```python
from build123d import *

# Parameters (mm, degrees)
SKETCH1_W           = 25
SKETCH1_H           = 25
SKETCH1_W_2         = 23
SKETCH1_H_2         = 23
BOSS_EXTRUDE1_DEPTH = 450
SKETCH2_W           = 25
SKETCH2_H           = 25
SKETCH2_W_2         = 23
SKETCH2_H_2         = 23
BOSS_EXTRUDE2_DEPTH = 200
SKETCH3_W           = 25
SKETCH3_H           = 25
SKETCH3_W_2         = 23
SKETCH3_H_2         = 23
BOSS_EXTRUDE3_DEPTH = 200
SKETCH4_W           = 25
SKETCH4_H           = 25
SKETCH4_W_2         = 23
SKETCH4_H_2         = 23
BOSS_EXTRUDE4_DEPTH = 125
SKETCH5_W           = 25
SKETCH5_H           = 25
SKETCH5_W_2         = 23
SKETCH5_H_2         = 23
BOSS_EXTRUDE5_DEPTH = 50
SKETCH6_R           = 2
CUT_EXTRUDE1_DEPTH  = 25
SKETCH7_W           = 25
SKETCH7_H           = 25
SKETCH7_W_2         = 23
SKETCH7_H_2         = 23
BOSS_EXTRUDE6_DEPTH = 125
SKETCH8_W           = 25
SKETCH8_H           = 25
SKETCH8_W_2         = 23
SKETCH8_H_2         = 23
BOSS_EXTRUDE7_DEPTH = 400


with BuildPart() as part:
    # Sketch1 → Boss-Extrude1 (new body)
    with BuildSketch(Plane.XY):
        Rectangle(SKETCH1_W, SKETCH1_H)
        Rectangle(SKETCH1_W_2, SKETCH1_H_2, mode=Mode.SUBTRACT)
    boss_extrude1 = extrude(amount=BOSS_EXTRUDE1_DEPTH)

    # Sketch2 → Boss-Extrude2 (add)
    with BuildSketch(Plane(origin=(12.5, 0, 0), x_dir=(0, 0, -1), z_dir=(1, 0, 0))):
        with Locations((-437.5, 0)):
            Rectangle(SKETCH2_W, SKETCH2_H)
        with Locations((-437.5, 0)):
            Rectangle(SKETCH2_W_2, SKETCH2_H_2, mode=Mode.SUBTRACT)
    boss_extrude2 = extrude(amount=BOSS_EXTRUDE2_DEPTH)

    # Sketch3 → Boss-Extrude3 (add)
    with BuildSketch(Plane(origin=(12.5, 0, 0), x_dir=(0, 0, -1), z_dir=(1, 0, 0))):
        with Locations((-12.5, 0)):
            Rectangle(SKETCH3_W, SKETCH3_H)
        with Locations((-12.5, 0)):
            Rectangle(SKETCH3_W_2, SKETCH3_H_2, mode=Mode.SUBTRACT)
    boss_extrude3 = extrude(amount=BOSS_EXTRUDE3_DEPTH)

    # Mirror1: Boss-Extrude1, Boss-Extrude2, Boss-Extrude3 across plane
    add(boss_extrude1.mirror(Plane(origin=(212.5, 0, 0), x_dir=(0, 0, 1), z_dir=(1, 0, 0))))
    add(boss_extrude2.mirror(Plane(origin=(212.5, 0, 0), x_dir=(0, 0, 1), z_dir=(1, 0, 0))))
    add(boss_extrude3.mirror(Plane(origin=(212.5, 0, 0), x_dir=(0, 0, 1), z_dir=(1, 0, 0))))

    # Sketch4 → Boss-Extrude4 (add)
    with BuildSketch(Plane(origin=(0, 12.5, 0), x_dir=(1, 0, 0), z_dir=(0, 1, 0))):
        with Locations((425, -187.5)):
            Rectangle(SKETCH4_W, SKETCH4_H)
        with Locations((425, -187.5)):
            Rectangle(SKETCH4_W_2, SKETCH4_H_2, mode=Mode.SUBTRACT)
    extrude(amount=BOSS_EXTRUDE4_DEPTH)

    # Sketch5 → Boss-Extrude5 (add)
    with BuildSketch(Plane.ZY.offset(-412.5)):
        with Locations((187.5, 125)):
            Rectangle(SKETCH5_W, SKETCH5_H)
        with Locations((187.5, 125)):
            Rectangle(SKETCH5_W_2, SKETCH5_H_2, mode=Mode.SUBTRACT)
    extrude(amount=BOSS_EXTRUDE5_DEPTH)

    # Sketch6 → Cut-Extrude1 (cut)
    with BuildSketch(Plane(origin=(0, 137.5, 0), x_dir=(1, 0, 0), z_dir=(0, 1, 0))):
        with Locations(Location((367.5, -180, 0), (0, 0, 270))):
            Circle(SKETCH6_R)
        with Locations(Location((367.5, -195, 0), (0, 0, 270))):
            Circle(SKETCH6_R)
        with Locations(Location((377.5, -180, 0), (0, 0, 270))):
            Circle(SKETCH6_R)
        with Locations(Location((377.5, -195, 0), (0, 0, 270))):
            Circle(SKETCH6_R)
        with Locations(Location((387.5, -180, 0), (0, 0, 270))):
            Circle(SKETCH6_R)
        with Locations(Location((387.5, -195, 0), (0, 0, 270))):
            Circle(SKETCH6_R)
    extrude(amount=-CUT_EXTRUDE1_DEPTH, mode=Mode.SUBTRACT)

    # Sketch7 → Boss-Extrude6 (add)
    # profile 1 of 2: a face of its own
    with BuildSketch(Plane(origin=(0, 12.5, 0), x_dir=(1, 0, 0), z_dir=(0, 1, 0))):
        with Locations((425, -437.5)):
            Rectangle(SKETCH7_W, SKETCH7_H)
        with Locations((425, -437.5)):
            Rectangle(SKETCH7_W_2, SKETCH7_H_2, mode=Mode.SUBTRACT)
    # profile 2 of 2: a face of its own
    with BuildSketch(Plane(origin=(0, 12.5, 0), x_dir=(1, 0, 0), z_dir=(0, 1, 0))):
        with Locations((0, -437.5)):
            Rectangle(SKETCH7_W, SKETCH7_H)
        with Locations((0, -437.5)):
            Rectangle(SKETCH7_W_2, SKETCH7_H_2, mode=Mode.SUBTRACT)
    extrude(amount=BOSS_EXTRUDE6_DEPTH)

    # Sketch8 → Boss-Extrude7 (add)
    with BuildSketch(Plane.ZY.offset(-412.5)):
        with Locations((437.5, 125)):
            Rectangle(SKETCH8_W, SKETCH8_H)
        with Locations((437.5, 125)):
            Rectangle(SKETCH8_W_2, SKETCH8_H_2, mode=Mode.SUBTRACT)
    extrude(amount=BOSS_EXTRUDE7_DEPTH)


solid = part.part
```
CAD build for the part. Positions are in the model's coordinates, mm. A direction names the side the tool comes from. Coordinates: 2 decimals unless noted, no trailing zeros. Write each loop counter-clockwise with the first axis right and the second up, starting at its lowest first coordinate (ties: lowest second). Pieces come first, ordered by that corner, then holes.
(1) Cut at D-D, the plane y = 72.5. List the corners of the cut face in (x, z), and give its area (3 significant figures).
(2) Drill centre lines: probe 1 along X at (y, z) = (112.8, 180); probe 2 along Z at (x, y) = (387, 137); probe 3 along Z at (x, y) = (296, 6.5). Where is each one in solid material? Low to high.
(3) Cut at C-C, the plane z = 342.5. List the corners of the cut face in (x, y), and give its area (3 significant figures).
(4) Two-plate mould, pull along X, no slides. Class faces 1 (the face through (215, 112.5, 437)), 2 (the face through (425, 74, 176)), 3 (the face through (-12.5, 12, 257)), 4 (the face through (388, 112.5, 187)): +X half, -X half, draft (parallel to the pull), parting line (faces both ways), or undercut.
(5) Flat gauge pins, fed straight in: pin 1 (11.5 mm diameter, centred on x = 427, z = 190.5, fed in from +Y); pin 2 (6.5 mm diameter, centred on x = 387.5, z = 195, fed in from -Y); pin 3 (18.5 mm diameter, centred on x = 420.5, y = 70, fed in from -Z). Where does each tip first touch, or does it go through?
(6) Cut at A-A, the plane x = 189. List the corners of the cut face in (y, z).
(7) Cut at B-B, the plane y = 125. List the corners of the cut face in (x, z), and give its area (3 significant figures).
(8) 3-axis set-ups, long thin cutter, end or side, ignore diameter. For faces 5 (the face through (413.5, 0, 222)), 6 (the face through (0, 74, 426)), 7 (the face through (215, 0, 449)): which of +Z, -Z, +X, -X, +Y, -Y reach the whole face in a straight line?
Geometry says:
1. outline: (-12.5, 425) - (12.5, 425) - (12.5, 450) - (-12.5, 450) - close; (412.5, 175) - (437.5, 175) - (437.5, 200) - (412.5, 200) - close; (412.5, 425) - (437.5, 425) - (437.5, 450) - (412.5, 450) - close; hole (-11.5, 426) - (11.5, 426) - (11.5, 449) - (-11.5, 449) - close; hole (413.5, 176) - (436.5, 176) - (436.5, 199) - (413.5, 199) - close; hole (413.5, 426) - (436.5, 426) - (436.5, 449) - (413.5, 449) - close
1. area: 288 mm2
2. probe 1: x = 362.5 to 365.5, 369.5 to 375.5, 379.5 to 385.5, 389.5 to 413.5, 436.5 to 437.5
2. probe 2: z = 175 to 178.06, 181.94 to 193.06, 196.94 to 200, 425 to 450
2. probe 3: z = 0 to 1, 24 to 25, 425 to 426, 449 to 450
3. outline: (-12.5, -12.5) - (12.5, -12.5) - (12.5, 12.5) - (-12.5, 12.5) - close; (412.5, -12.5) - (437.5, -12.5) - (437.5, 12.5) - (412.5, 12.5) - close; hole (-11.5, -11.5) - (11.5, -11.5) - (11.5, 11.5) - (-11.5, 11.5) - close; hole (413.5, -11.5) - (436.5, -11.5) - (436.5, 11.5) - (413.5, 11.5) - close
3. area: 192 mm2
4. face 1: undercut
4. face 2: undercut
4. face 3: -X half
4. face 4: draft
5. pin 1: stops at y = 12.5
5. pin 2: stops at y = 112.5
5. pin 3: stops at z = 175
6. outline: (-12.5, 0) - (12.5, 0) - (12.5, 25) - (-12.5, 25) - close; (-12.5, 425) - (12.5, 425) - (12.5, 450) - (-12.5, 450) - close; (112.5, 425) - (137.5, 425) - (137.5, 450) - (112.5, 450) - close; hole (-11.5, 1) - (11.5, 1) - (11.5, 24) - (-11.5, 24) - close; hole (-11.5, 426) - (11.5, 426) - (11.5, 449) - (-11.5, 449) - close; hole (113.5, 426) - (136.5, 426) - (136.5, 449) - (113.5, 449) - close
7. outline: (-12.5, 425) - (437.5, 425) - (437.5, 450) - (-12.5, 450) - close; (362.5, 175) - (437.5, 175) - (437.5, 200) - (362.5, 200) - (362.5, 199) - (412.5, 199) - (412.5, 176) - (362.5, 176) - close; hole (-11.5, 426) - (11.5, 426) - (11.5, 449) - (-11.5, 449) - close; hole (12.5, 426) - (412.5, 426) - (412.5, 449) - (12.5, 449) - close; hole (413.5, 176) - (436.5, 176) - (436.5, 199) - (413.5, 199) - close; hole (413.5, 426) - (436.5, 426) - (436.5, 449) - (413.5, 449) - close
7. area: 1,190 mm2
8. face 5: +Z, -Z
8. face 6: +Y
8. face 7: none
